Source: CAD feature listing. Evaluate the final solid. Frame: model axes, mm. Round coordinates to 2 decimals unless told otherwise and drop trailing zeros. Loops run counter-clockwise (first coordinate to the right, second up) from the corner with the lowest first, then second, coordinate; pieces in that order, holes last. Notation, with made-up numbers: M -8,47.25 L 3,47.25 A26 cw 3,79.25 Z; hole C 13.5,24.25 d9. An arc over 180 degrees is marked long. Write each question's results on one line, items separated by ' | '. Start each with the question number.
1. Section A-A on x = -83.82. Output: boundary loops of the cut face in (y, z), and give its area (3 significant figures).
2. Section B-B on y = 0. Output: boundary loops of the cut face in (x, z), and give its area (3 significant figures).
3. Contact query for flat-ended pins moving along their axis: pin 1 Ø4 at (x, y) = (-36, 0.5) entering from +Z; pin 2 Ø4 at (x, y) = (-84, -148.5) entering from -Z; pin 3 Ø7 at (x, z) = (-83.82, -7.62) entering from +Y. Output: stop coordinate, or through.
4. Section C-C on x = -38.1. Output: boundary loops of the cut face in (y, z).
5. Ray query, line 1 (Y direction, x = 38.1, z = -1.1); line 2 (X direction, y = 153.25, z = -7.62); line 3 (X direction, y = -5, z = -4). Return the intervals inside material, ascending.
from build123d import *

# Parameters (mm, degrees)
SKETCH1_W           = 180.34
SKETCH1_H           = 314.96
BOSS_EXTRUDE1_DEPTH = 12.7
SKETCH4_R           = 6.35
CUT_EXTRUDE2_DEPTH  = 5.08
SKETCH6_R           = 3.81
CUT_EXTRUDE3_DEPTH  = 5.08
SKETCH7_R           = 3.81
CUT_EXTRUDE4_DEPTH  = 7.62
SKETCH8_R           = 3.81
CUT_EXTRUDE5_DEPTH  = 7.62


with BuildPart() as part:
    # Sketch1 → Boss-Extrude1 (new body)
    with BuildSketch(Plane.XY):
        Rectangle(SKETCH1_W, SKETCH1_H)
    extrude(amount=-BOSS_EXTRUDE1_DEPTH)

    # Sketch4 → Cut-Extrude2 (cut)
    with BuildSketch(Plane.XY):
        with Locations((-38.1, 0)):
            Circle(SKETCH4_R)
        with Locations((38.1, 0)):
            Circle(SKETCH4_R)
    extrude(amount=-CUT_EXTRUDE2_DEPTH, mode=Mode.SUBTRACT)

    # Sketch6 → Cut-Extrude3 (cut)
    with BuildSketch(Plane(origin=(0, 0, -12.7), x_dir=(-1, 0, 0), z_dir=(0, 0, -1))):
        with Locations((83.759872632, 149.86)):
            Circle(SKETCH6_R)
        with Locations((83.82, -149.86)):
            Circle(SKETCH6_R)
    extrude(amount=-CUT_EXTRUDE3_DEPTH, mode=Mode.SUBTRACT)

    # Sketch7 → Cut-Extrude4 (cut)
    with BuildSketch(Plane(origin=(0, 157.48, 0), x_dir=(1, 0, 0), z_dir=(0, 1, 0))):
        with Locations((-83.82, 7.62)):
            Circle(SKETCH7_R)
    extrude(amount=-CUT_EXTRUDE4_DEPTH, mode=Mode.SUBTRACT)

    # Sketch8 → Cut-Extrude5 (cut)
    with BuildSketch(Plane(origin=(0, -157.48, 0), x_dir=(-1, 0, 0), z_dir=(0, -1, 0))):
        with Locations((83.82, 7.62)):
            Circle(SKETCH8_R)
    extrude(amount=-CUT_EXTRUDE5_DEPTH, mode=Mode.SUBTRACT)


solid = part.part
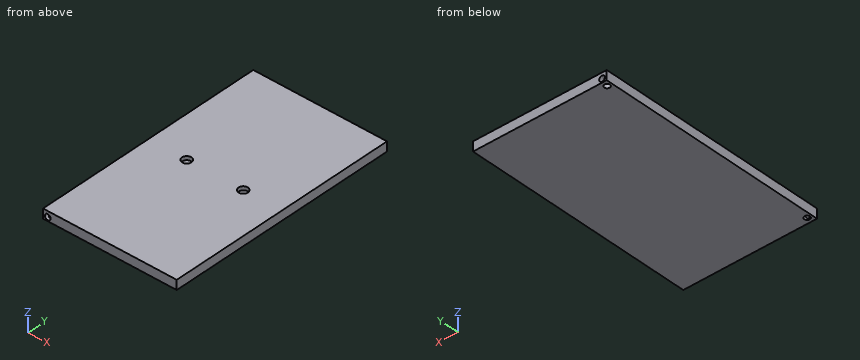
Taken from the geometry:
1) outline: M -157.48,-12.7 L -153.67,-12.7 L -153.67,-11.43 L -157.48,-11.43 Z; M -157.48,-3.81 L -149.86,-3.81 L -149.86,-7.62 L -146.05,-7.62 L -146.05,-12.7 L 146.05,-12.7 L 146.05,-7.62 L 149.86,-7.62 L 149.86,-3.81 L 157.48,-3.81 L 157.48,0 L -157.48,0 Z; M 153.67,-12.7 L 157.48,-12.7 L 157.48,-11.43 L 153.67,-11.43 Z | area: 3,840 mm^2
2) outline: M -90.17,-12.7 L 90.17,-12.7 L 90.17,0 L 44.45,0 L 44.45,-5.08 L 31.75,-5.08 L 31.75,0 L -31.75,0 L -31.75,-5.08 L -44.45,-5.08 L -44.45,0 L -90.17,0 Z | area: 2,160 mm^2
3) pin 1: z = -5.08 | pin 2: z = -7.62 | pin 3: y = 149.86
4) outline: M -157.48,-12.7 L 157.48,-12.7 L 157.48,0 L 6.35,0 L 6.35,-5.08 L -6.35,-5.08 L -6.35,0 L -157.48,0 Z
5) line 1: -157.48 to -6.35, 6.35 to 157.48 | line 2: -90.17 to -87.63, -80.01 to 90.17 | line 3: -90.17 to -42.01, -34.19 to 34.19, 42.01 to 90.17
